Could you check a few things on this model? Use its own coordinates, in mm. A direction names the side the tool comes from. Coordinates: 2 decimals unless noted, no trailing zeros. Loops run counter-clockwise (first coordinate to the right, second up) from the corner with the lowest first, then second, coordinate; pieces in that order, holes last. Notation, with made-up numbers: (15.25, 42) - (45.25, 42) arc R11 cw to (45.25, 57) - close; hole circle Ø7 at (-21.75, -5). An arc over 180 degrees is marked (long way). One line per item, written item: value. Start each with the question number.
(1) If we mould it in two halves opening along Z, with no side actions, what happens to faces 3 (the face through (-22, 0, -38)), 4 (the face through (-23, 3, 22.43)), 5 (the face through (-4.17, 1.67, 7.42))? For each: pulls with the +Z half, pulls with the -Z half, needs draft (parallel to the pull), parting line crosses it, or undercut.
(2) If we section it at C-C on z = -76: Write out the boundary of the cut face in (x, y), then the cut area to 3 significant figures.
(3) I'm going to push flat-ended pins straight in: P1, Ø4.5, axis at x = -2.6, z = -27.57, coming from the -Y side; P2, Ø8, axis at x = -42.71, z = 12.43, coming from the -Y side. Where does each tip first touch, or does it pass through?
(4) If we section it at B-B on z = -59: Write out the boundary of the cut face in (x, y).
(5) On a 3-axis mill with a long thin cutter (end or side, diameter ignored), from which of +Z, -Z, +X, -X, +Y, -Y can I reach the whole of each face in a straight line? I mean faces 1 (the face through (0, 3.3, -29)), 2 (the face through (-62.654, 3, -38)). Say none if no direction works.
(6) If we section it at A-A on x = -10: Write out the boundary of the cut face in (y, z), then the cut area to 3 significant figures.
(7) If we section it at D-D on y = 1.5: Write out the boundary of the cut face in (x, z), then the cut area to 3 significant figures.
(8) If I drill on line 1 along Z through (x, y) = (-43, 4.2); line 2 along Z through (x, y) = (7.5, 0.3); line 3 along Z through (x, y) = (-24.5, 3.7), over which ranges is the centre line in solid material (lowest first)? Write a range as from..to.
Autodesk Inventor part; units mm, degrees
ref_plane "YZ Plane" through (0, 0, 0) normal (1, 0, 0) x (0, 1, 0)
ref_plane "XZ Plane" through (0, 0, 0) normal (0, 1, 0) x (-1, 0, 0)
ref_plane "XY Plane" through (0, 0, 0) normal (0, 0, 1) x (1, 0, 0)
sketch "Schizzo1" plane through (0, 0, 0) normal (0, 1, 0) x (-1, 0, 0)
  line L0 (87.6536, 7.4302) -> (-32.3464, 7.4302)
  line L1 (-32.3464, 7.4302) -> (-32.3464, -72.5698)
  line L2 (-32.3464, -72.5698) -> (87.6536, -72.5698)
  line L3 (87.6536, -72.5698) -> (87.6536, 7.4302)
  point P0 (0, 0)
  dimension "d0" = 80
  dimension "d1" = 120
extrude "Estrusione1" add sketch "Schizzo1" along normal blind 6
move or copy body "Sposta corpo1" bodies to move or copy 1 copy no rotation origin (0, 0, 0) rotation axis (0, 1, 0) rotation angle 90 translate (9.9162, 0, -65.2235)
sketch "Schizzo7" plane through (-62.6536, 0, -97.5698) normal (0, -1, 0) x (1, 0, 0)
  circle A0 centre (19.9435, 110) radius 4
  circle A1 centre (19.9435, 70) radius 4
  circle A2 centre (60.0565, 70) radius 4
  circle A3 centre (60.0565, 110) radius 4
hole "Foro1" at (-2.5971, 0, 12.4302) at (-2.5971, 0, -27.5698) at (-42.7101, 0, -27.5698) at (-42.7101, 0, 12.4302) direction (0, 1, 0) diameter 4.917 end through all counterbore diameter 10.5 counterbore depth 3.3
sketch "Schizzo8" plane through (-62.6536, 0, -97.5698) normal (0, -1, 0) x (1, 0, 0)
  line L0 (75.3545, 58.287) -> (35.3545, 58.287)
  line L1 (35.3545, 58.287) -> (35.3545, 18.287)
  line L2 (35.3545, 18.287) -> (75.3545, 18.287)
  line L3 (75.3545, 18.287) -> (75.3545, 58.287)
  circle A0 centre (55.3545, 38.287) radius 15
  circle A1 centre (39.0911, 54.5505) radius 2.25
  circle A2 centre (71.618, 54.5505) radius 2.25
  circle A3 centre (39.0911, 22.0236) radius 2.25
  circle A4 centre (71.618, 22.0236) radius 2.25
  point P0 (62.6536, 97.5698)
  dimension "d14" = 30
  dimension "d16" = 4.5
  dimension "d17" = 4.5
  dimension "d18" = 4.5
  dimension "d19" = 4.5
hole "Foro2" at (8.9643, 0, -43.0193) direction (0, 1, 0) diameter 3.9587 depth 6
hole "Foro3" at (-23.5626, 0, -43.0193) direction (0, 1, 0) diameter 3.9587 depth 6
hole "Foro4" at (-23.5626, 0, -75.5463) direction (0, 1, 0) diameter 3.9587 depth 6
hole "Foro5" at (8.9643, 0, -75.5463) direction (0, 1, 0) diameter 3.9587 depth 6
sketch "Schizzo9" plane through (-62.6536, 0, -97.5698) normal (0, -1, 0) x (1, 0, 0)
  line L0 (35.3545, 58.287) -> (75.3545, 58.287)
  line L1 (75.3545, 58.287) -> (75.3545, 18.287)
  line L2 (75.3545, 18.287) -> (35.3545, 18.287)
  line L3 (35.3545, 18.287) -> (35.3545, 58.287)
  point P0 (62.6536, 97.5698)
  point P1 (35.3545, 18.287)
  point P2 (75.3545, 58.287)
  point P3 (55.3545, 38.287)
extrude "Estrusione2" cut sketch "Schizzo9" against normal blind 3
hole "Foro6" at (-7.2991, 0, -59.2828) direction (0, 1, 0) diameter 30 depth 6
equation "\"RaggioPiega\" = Spessore"
equation "\"LarghezzaScaricoPiega\" = Spessore"
equation "\"ProfonditàScaricoPiega\" = 0.5 * Spessore"
equation "\"DimensioniScaricoAngolo\" = 4 * Spessore"
equation "\"ResiduoMinimo\" = 2 * Spessore"
equation "\"RaggioTransizione\" = RaggioPiega"
equation "\"Dimensione_raggio_Jacobi\" = RaggioPiega"
equation "\"DimensioneGioco\" = Spessore"
properties part number "Platform"
Values:
1. face 3: needs draft
1. face 4: pulls with the +Z half
1. face 5: undercut
2. outline: (-62.65, 0) - (-27.3, 0) - (-27.3, 3) - (-25.49, 3) - (-25.49, 6) - (-62.65, 6) - close; (-21.64, 3) - (7.04, 3) - (7.04, 6) - (-21.64, 6) - close; (10.89, 3) - (12.7, 3) - (12.7, 0) - (17.35, 0) - (17.35, 6) - (10.89, 6) - close
2. area: 337 mm2
3. P1: passes through
3. P2: stops at y = 3.3
4. outline: (-62.65, 0) - (-27.3, 0) - (-27.3, 3) - (-22.3, 3) - (-22.3, 6) - (-62.65, 6) - close; (7.7, 3) - (12.7, 3) - (12.7, 0) - (17.35, 0) - (17.35, 6) - (7.7, 6) - close
5. face 1: -Y
5. face 2: +Z, -Z, -X, +Y, -Y
6. outline: (0, -97.57) - (6, -97.57) - (6, -74.04) - (3, -74.04) - (3, -79.28) - (0, -79.28) - close; (0, -39.28) - (3, -39.28) - (3, -44.53) - (6, -44.53) - (6, 22.43) - (0, 22.43) - close
6. area: 511 mm2
7. outline: (-62.65, -97.57) - (17.35, -97.57) - (17.35, 22.43) - (-62.65, 22.43) - close; hole circle Ø10.5 at (-42.71, -27.57); hole circle Ø10.5 at (-42.71, 12.43); hole (-27.3, -79.28) - (12.7, -79.28) - (12.7, -39.28) - (-27.3, -39.28) - close; hole circle Ø10.5 at (-2.6, -27.57); hole circle Ø10.5 at (-2.6, 12.43)
7. area: 7,650 mm2
8. line 1: z = -97.57..-30.01, -25.13..9.99, 14.87..22.43
8. line 2: z = -97.57..-79.28, -39.28..22.43
8. line 3: z = -97.57..-77.29, -73.8..-44.76, -41.28..22.43
